Autodesk Inventor part; units mm, degrees
ref_plane "YZ Plane" through (0, 0, 0) normal (1, 0, 0) x (0, 1, 0)
ref_plane "XZ Plane" through (0, 0, 0) normal (0, 1, 0) x (-1, 0, 0)
ref_plane "XY Plane" through (0, 0, 0) normal (0, 0, 1) x (1, 0, 0)
sketch "Esboço1" plane through (0, 0, 0) normal (0, 0, 1) x (1, 0, 0)
  line L0 (-29.0921, 25.5754) -> (20.9079, 25.5754)
  line L1 (20.9079, 25.5754) -> (20.9079, -54.4246)
  line L2 (20.9079, -54.4246) -> (-29.0921, -54.4246)
  line L3 (-29.0921, -54.4246) -> (-29.0921, 25.5754)
  point P0 (0, 0)
extrude "Extrusão1" add sketch "Esboço1" along normal blind 10
fillet "Arredondamento1" radius 10 4 edges at (-29.0921, 25.5754, 5) (20.9079, 25.5754, 5) (20.9079, -54.4246, 5) (-29.0921, -54.4246, 5)
fillet "Arredondamento2" radius 4 8 edges at (-26.1631, 22.6465, 0) (-29.0921, -14.4246, 0) (-26.1631, -51.4956, 0) (-4.0921, -54.4246, 0) (17.979, -51.4956, 0) (20.9079, -14.4246, 0) (17.979, 22.6465, 0) (-4.0921, 25.5754, 0)
shell "Casca1" thickness 2 removed faces 1 at (-12.4254, -4.4246, 10)
sketch "Esboço2" plane through (-19.0921, -50.4246, 2) normal (0, 0, 1) x (1, 0, 0)
  arc A0 (-8, 6) -> (0, -2) centre (0, 6) ccw
  line L0 (-8, 6) -> (-8, 66)
  arc A1 (0, 74) -> (-8, 66) centre (0, 66) ccw
  line L1 (0, 74) -> (30, 74)
  arc A2 (38, 66) -> (30, 74) centre (30, 66) ccw
  line L2 (38, 66) -> (38, 6)
  arc A3 (30, -2) -> (38, 6) centre (30, 6) ccw
  line L3 (30, -2) -> (0, -2)
  arc A4 (-10, 6) -> (0, -4) centre (0, 6) ccw
  line L4 (0, -4) -> (30, -4)
  arc A5 (30, -4) -> (40, 6) centre (30, 6) ccw
  line L5 (40, 6) -> (40, 66)
  arc A6 (40, 66) -> (30, 76) centre (30, 66) ccw
  line L6 (30, 76) -> (0, 76)
  arc A7 (0, 76) -> (-10, 66) centre (0, 66) ccw
  line L7 (-10, 66) -> (-10, 6)
  arc A8 (0, 72) -> (-6, 66) centre (0, 66) ccw
  circle A9 centre (2, 64) radius 2
  circle A10 centre (28, 64) radius 2
  circle A11 centre (2, 24) radius 2
  circle A12 centre (28, 24) radius 2
  point P0 (19.0921, 50.4246)
  dimension "d16" = 8
  dimension "d17" = 8
  dimension "d18" = 36
  dimension "d19" = 36
  dimension "d20" = 12
  dimension "d21" = 12
extrude "Extrusão2" add sketch "Esboço2" along normal up to surface (8 mm away) contours A9 | A10 | A11 | A12
equation "\"d17\" = d16"
equation "\"d19\" = d18"
properties part number "Carcaca-Baixa"
Geometry check sheet. Reference: the model listing, model coordinates, mm. A direction names the side the tool comes from. Give positions to 0.01 mm unless a question says otherwise; leave off trailing zeros. Write each loop counter-clockwise with the first axis right and the second up, starting at its lowest first coordinate (ties: lowest second). Pieces come first, ordered by that corner, then holes.
1) Thickness scan on line 1 (Y direction, x = 9, z = 9); line 2 (Y direction, x = 1, z = 8.75); line 3 (X direction, y = -1.5, z = 5). Record the ranges inside material, lowest first.
Values follow:
line 1: y = -54.42 to -52.42, -28.42 to -24.43, 11.58 to 15.57, 23.58 to 25.58
line 2: y = -54.42 to -52.42, 23.58 to 25.58
line 3: x = -29.09 to -27.09, 18.91 to 20.91
2) Cross-section at C-C (y = -1.5). Record the boundary of the cut face in (x, z).
Values follow:
outline: (-29.09, 4) arc R4 ccw to (-25.09, 0) - (16.91, 0) arc R4 ccw to (20.91, 4) - (20.91, 10) - (18.91, 10) - (18.91, 4) arc R2 cw to (16.91, 2) - (-25.09, 2) arc R2 cw to (-27.09, 4) - (-27.09, 10) - (-29.09, 10) - close
3) Cross-section at A-A (z = 8). Record the boundary of the cut face in (x, y).
Values follow:
outline: (-29.09, -44.42) arc R10 ccw to (-19.09, -54.42) - (10.91, -54.42) arc R10 ccw to (20.91, -44.42) - (20.91, 15.58) arc R10 ccw to (10.91, 25.58) - (-19.09, 25.58) arc R10 ccw to (-29.09, 15.58) - close; circle Ø4 at (-17.09, -26.42); circle Ø4 at (-17.09, 13.58); circle Ø4 at (8.91, -26.42); circle Ø4 at (8.91, 13.58); hole (-27.09, -44.42) arc R8 ccw to (-19.09, -52.42) - (10.91, -52.42) arc R8 ccw to (18.91, -44.42) - (18.91, 15.58) arc R8 ccw to (10.91, 23.58) - (-19.09, 23.58) arc R8 ccw to (-27.09, 15.58) - close
4) Cross-section at B-B (x = 6). Record the boundary of the cut face in (y, z).
Values follow:
outline: (-54.42, 4) arc R4 ccw to (-50.42, 0) - (21.58, 0) arc R4 ccw to (25.58, 4) - (25.58, 10) - (23.58, 10) - (23.58, 4) arc R2 cw to (21.58, 2) - (-50.42, 2) arc R2 cw to (-52.42, 4) - (-52.42, 10) - (-54.42, 10) - close
5) Cross-section at D-D (x = -17). Record the boundary of the cut face in (y, z), plus the area to 3 significant figures.
Values follow:
outline: (-54.42, 4) arc R4 ccw to (-50.42, 0) - (21.58, 0) arc R4 ccw to (25.58, 4) - (25.58, 10) - (23.58, 10) - (23.58, 4) arc R2 cw to (21.58, 2) - (15.57, 2) - (15.57, 10) - (11.58, 10) - (11.58, 2) - (-24.43, 2) - (-24.43, 10) - (-28.42, 10) - (-28.42, 2) - (-50.42, 2) arc R2 cw to (-52.42, 4) - (-52.42, 10) - (-54.42, 10) - close
area: 251 mm2
6) Go/stop test with a flat-tipped pin: pin 1 Ø12.5 at (x, y) = (0.5, -6.5) entering from +Z. Record where the tip stops, or that it passes through.
Values follow:
pin 1: stops at z = 2
7) Release check for a two-part mould opening along X. For faces 3 (the face through (-4, 25.575, 7)), 4 (the face through (-4.302, 23.005, 2.601)), 5 (the face through (19.767, -14.005, 1.203)) record: released by +X, released by -X, zero draft, split by the parting line, or undercut.
Values follow:
face 3: zero draft
face 4: undercut
face 5: released by +X
8) Set-up check for faces 1 (the face through (-3.882, -51.854, 2.601)), 2 (the face through (-28, -14, 10)): record each of +Z, -Z, +X, -X, +Y, -Y from which the full face is reachable in a straight line by a thin tool's end or side.
Values follow:
face 1: +Z
face 2: +Z, +X, -X, +Y, -Y
